Part model, mm, in its own coordinate system. Face numbers are marked on the shaded views. A direction names the side the tool comes from. Give positions to 0.01 mm unless a question says otherwise; leave off trailing zeros. Write each loop counter-clockwise with the first axis right and the second up, starting at its lowest first coordinate (ties: lowest second). Pieces come first, ordered by that corner, then holes.
from build123d import *

# Parameters (mm, degrees)
F1_DEPTH = 12.5
F2_W     = 11
F2_H     = 7
F3_DEPTH = 14.001


with BuildPart() as f1:
    # F0 (on Right) → F1 (new body, symmetric)
    with BuildSketch(Plane.YZ):
        Polygon((-11, 14), (-11, 0), (0, 0), (0, 9), (14, 9), (14, 25), (4, 25), (4, 14), align=None)
    extrude(amount=F1_DEPTH, both=True)

    # F2 (on face) → F3 (cut, through all)
    with BuildSketch(Plane.XY.offset(14)):
        with Locations((0, -7.5)):
            Rectangle(F2_W, F2_H)
    extrude(amount=-F3_DEPTH, mode=Mode.SUBTRACT)


solid = f1.part
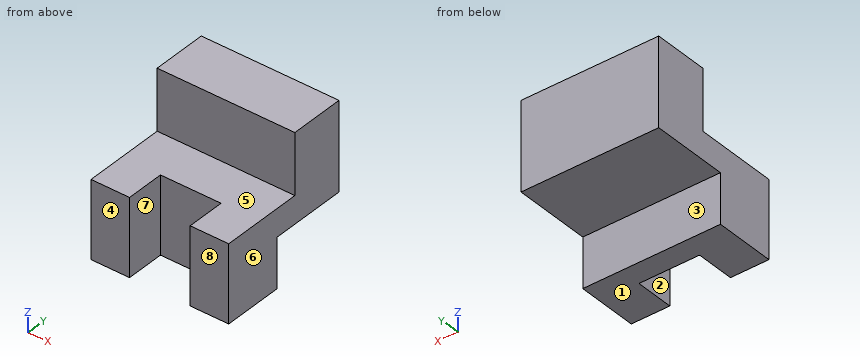
1) Drill centre lines: L1, parallel to Y at x = -11, z = 8.5; L2, parallel to Z at x = -3.75, y = 11.5; L3, parallel to X at y = -6, z = 2. Where is each one in solid material? Low to high.
Check result:
L1: y = -11 to 0
L2: z = 9 to 25
L3: x = -12.5 to -5.5, 5.5 to 12.5
2) Flat gauge pins, fed straight in: P1, Ø5, axis at x = 6.5, y = -8.5, coming from the -Z side; P2, Ø1, axis at x = 7, z = 7.5, coming from the +Y side; P3, Ø3, axis at x = 3, y = -0.5, coming from the +Z side; P4, Ø4, axis at x = 0.5, y = 10.5, coming from the -Z side. Where does each tip first touch, or does it go through?
Check result:
P1: stops at z = 0
P2: stops at y = 0
P3: stops at z = 14
P4: stops at z = 9
3) Mould opens along X. For the marked faces 6, 7 and 8 say: +X half, -X half, draft (parallel to the pull), parting line (faces both ways), or undercut.
Check result:
face 6: +X half
face 7: undercut
face 8: draft
4) Saw through at D-D (y = 0.75). Write the cut outline in (x, z), and give its area (3 significant figures).
Check result:
outline: (-12.5, 9) - (12.5, 9) - (12.5, 14) - (-12.5, 14) - close
area: 125 mm2
5) Saw through at C-C (z = 7.75). Write the cut outline in (x, y).
Check result:
outline: (-12.5, -11) - (-5.5, -11) - (-5.5, -4) - (5.5, -4) - (5.5, -11) - (12.5, -11) - (12.5, 0) - (-12.5, 0) - close
6) Saw through at B-B (y = -8). Write the cut outline in (x, z), and give its area (3 significant figures).
Check result:
outline: (-12.5, 0) - (-5.5, 0) - (-5.5, 14) - (-12.5, 14) - close; (5.5, 0) - (12.5, 0) - (12.5, 14) - (5.5, 14) - close
area: 196 mm2
7) Saw through at A-A (x = 3). Write the cut outline in (y, z), and give its area (3 significant figures).
Check result:
outline: (-4, 0) - (0, 0) - (0, 9) - (14, 9) - (14, 25) - (4, 25) - (4, 14) - (-4, 14) - close
area: 236 mm2
8) 3-axis set-ups, long thin cutter, end or side, ignore diameter. For the marked faces 1, 2, 3, 4 and 5: which of +Z, -Z, +X, -X, +Y, -Y reach the whole face in a straight line?
Check result:
face 1: -Z, +X, -X, +Y, -Y
face 2: +Z, -Z, -Y
face 3: -Z, +X, -X, +Y
face 4: +Z, -Z, +X, -X, -Y
face 5: +Z, +X, -X, -Y
